Geometry check sheet. Reference: the model listing, model coordinates, mm. Face numbers are marked on the shaded views. A direction names the side the tool comes from. Give positions to 0.01 mm unless a question says otherwise; leave off trailing zeros. Write each loop counter-clockwise with the first axis right and the second up, starting at its lowest first coordinate (ties: lowest second). Pieces come first, ordered by that corner, then holes. Notation, with made-up numbers: M 39.5,-26.5 L 56.5,-26.5 A13 cw 56.5,-3.5 Z; hole C -37.5,4 d11. An arc over 180 degrees is marked long. One line per item, written item: value. Start each with the question number.
1. Gauge pin test, flat ends, axial feed: pin 1 (1 mm diameter, centred on x = -1, y = 2, fed in from -Z); pin 2 (2 mm diameter, centred on x = -2, z = -18.5, fed in from -Y); pin 3 (1.5 mm diameter, centred on y = 0, z = -8, fed in from -X). Record the tip position at first contact, or that the pin passes through.
2. Cross-section at A-A on z = -8. Record the cut outline in (x, y).
3. Tool access check on the marked faces 1 and 2. Record the directions out of +Z, -Z, +X, -X, +Y, -Y that give a thin tool (end or side, any length) a straight path to the whole face; none if there is none.
4. Scan lines: line 1 (Z direction, x = -1.5, y = -2); line 2 (Y direction, x = 0, z = -6); line 3 (Y direction, x = -0.25, z = -1.5). Record each from-to range of solid material in increasing order.
Solid Edge part; units mm, degrees
sketch "Sketch1" plane through (0, 0, 0) normal (0, -1, 0) x (1, 0, 0)
  line L0 (0, 0) -> (2.8, 0)
  arc A0 (2.8, 0) -> (3.5, -0.7) centre (2.8, -0.7) cw
  line L1 (3.5, -0.7) -> (3.5, -4)
  line L2 (3.5, -4) -> (2, -4)
  line L3 (2, -4) -> (2, -33.3)
  line L4 (2, -33.3) -> (1.3, -34)
  line L5 (1.3, -34) -> (0, -34)
revolve "RevolvedProtrusion1" add sketch "Sketch1" angle 360 about axis through (0, 0, -34) along (0, 0, 1)
sketch "Sketch2" plane through (0, 0, 0) normal (0, 0, 1) x (1, 0, 0)
  line L0 (-1.5, -0.866) -> (-1.5, 0.866)
  line L1 (-1.5, 0.866) -> (0, 1.7321)
  line L2 (0, 1.7321) -> (1.5, 0.866)
  line L3 (1.5, 0.866) -> (1.5, -0.866)
  line L4 (1.5, -0.866) -> (0, -1.7321)
  line L5 (0, -1.7321) -> (-1.5, -0.866)
extrude "Cutout1" cut sketch "Sketch2" against normal blind 2
sketch "Sketch3" plane through (0, 0, 0) normal (1, 0, 0) x (0, 1, 0)
  line L0 (0, -3) -> (1.7321, -2)
  line L1 (0, -2) -> (1.7321, -2)
  line L2 (0, -2) -> (0, -3)
revolve "RevolvedCutout1" cut sketch "Sketch3" angle 360 about axis through (0, 0, -60.325) along (0, 0, 1)
cosmetic_thread "Thread1"
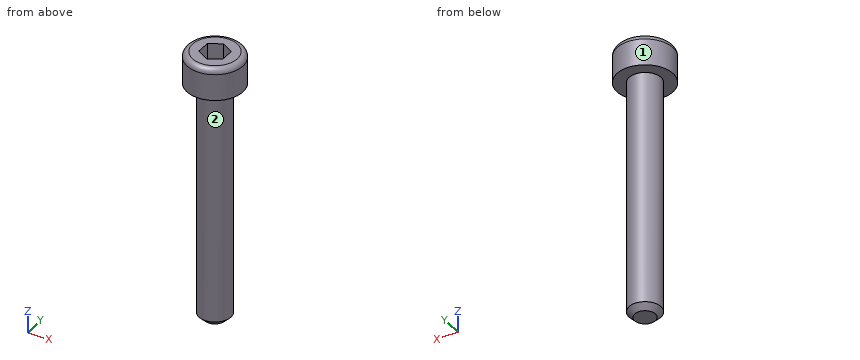
Report:
1. pin 1: stops at z = -33.56
1. pin 2: stops at y = -1.73
1. pin 3: stops at x = -2
2. outline: C 0,0 d4
3. face 1: +Z, -Z
3. face 2: -Z
4. line 1: z = -4 to 0
4. line 2: y = -2 to 2
4. line 3: y = -3.49 to -1.59, 1.59 to 3.49
